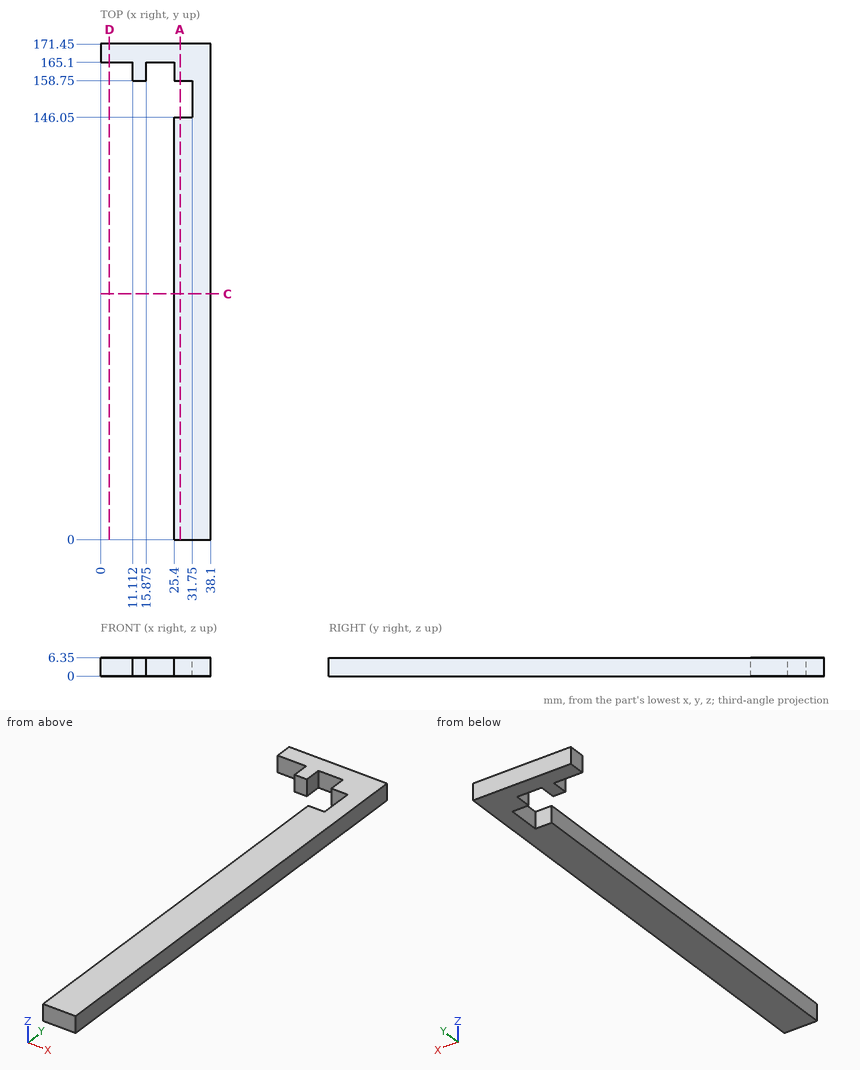
Study the drawing (mm; zero at the part's minimum x, y, z) and answer. Give positions to 0.01 mm unless a question says otherwise; leave off trailing zeros. Write each loop counter-clockwise with the first axis right and the second up, starting at its lowest first coordinate (ties: lowest second). Pieces come first, ordered by that corner, then holes. Notation, with made-up numbers: (-40, -20.5) - (-9, -20.5) arc R3 ccw to (-9, -16.5) - close; hole circle Ø7 at (69.5, 55). An arc over 180 degrees is marked (long way). One line per question, with ' | ' between items. Start each with the question number.
1. Straight lines are drawn through the part: line 1 (X direction, y = 110, z = 3.75); line 2 (X direction, y = 156.5, z = 4.75); line 3 (Y direction, x = 18.5, z = 6). For each, find the intervals that lie inside material, in ascending order.
2. Given P1, Ø2, axis at x = 4.5, z = 2, coming from the -Y side; P2, Ø1.9, axis at y = 152.5, z = 3, coming from the -X side, each flat-ended and moving along its own axis, determine where each tip first touches the part or whether it passes through.
3. Section A-A, the plane x = 27.5 is taken. Determine the outline of the cut face in (y, z).
4. Section C-C, the plane y = 85 is taken. Determine the outline of the cut face in (x, z).
5. Section D-D, the plane x = 3 is taken. Determine the outline of the cut face in (y, z).
Result:
1) line 1: x = 25.4 to 38.1 | line 2: x = 31.75 to 38.1 | line 3: y = 165.1 to 171.45
2) P1: stops at y = 165.1 | P2: stops at x = 31.75
3) outline: (0, 0) - (146.05, 0) - (146.05, 6.35) - (0, 6.35) - close; (158.75, 0) - (171.45, 0) - (171.45, 6.35) - (158.75, 6.35) - close
4) outline: (25.4, 0) - (38.1, 0) - (38.1, 6.35) - (25.4, 6.35) - close
5) outline: (165.1, 0) - (171.45, 0) - (171.45, 6.35) - (165.1, 6.35) - close
